Geometry: final body of the model. Coordinates: model frame, mm. Give positions to 0.01 mm unless a question says otherwise; leave off trailing zeros. Order: outer loops, then holes, each group sorted by start corner. A loop starts at its lowest first (then second) coordinate and runs counter-clockwise, first axis right, second up. Notation, with made-up numbers: M 29.25,-27 L 66.25,-27 A20 ccw 66.25,-9 Z; hole C 86.25,71 d5. An arc over 180 degrees is marked long. Use CSV: the item, a comma, the result in double quotes.
```python
from build123d import *

# Parameters (mm, degrees)
F0_W     = 2225
F0_H     = 100
F1_DEPTH = 125
F2_SIZE2 = 40
F2_SIZE  = 85


with BuildPart() as f1:
    # F0 (on Front) → F1 (new body)
    with BuildSketch(Plane.XZ):
        with Locations((-1112.5, -50)):
            Rectangle(F0_W, F0_H)
    extrude(amount=F1_DEPTH)

    # F2
    f2_edges = [f1.edges().sort_by_distance(p)[0] for p in [
        (-1112.5, -125, 0),
        (-2225, -62.5, 0),
    ]]
    f2_side = f1.faces().sort_by_distance((-1112.5, -62.5, 0))[0]
    chamfer(f2_edges, length=F2_SIZE, length2=F2_SIZE2, reference=f2_side)


solid = f1.part
```
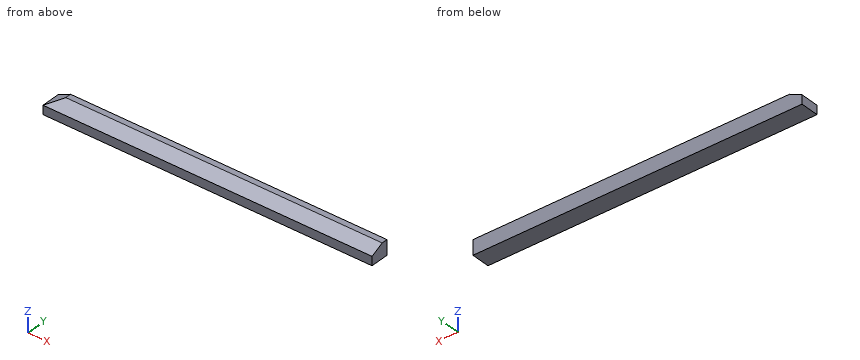
1. Section A-A, the plane x = -1465. Return the cut outline in (y, z).
Answer:
outline,"M -125,-100 L 0,-100 L 0,0 L -40,0 L -125,-40 Z"
2. Section B-B, the plane y = -87.5. Return the cut outline in (x, z), plus the area to 3 significant figures.
Answer:
outline,"M -2225,-100 L 0,-100 L 0,-22.35 L -2187.5,-22.35 L -2225,-40 Z"
area,"172,000 mm2"
3. Pin query (flat end, axial travel): pin 1 Ø1.5 at (x, y) = (-504.5, -109.5) entering from +Z; pin 2 Ø2 at (x, y) = (-1320.5, -83.5) entering from +Z. Return the tip coordinate at first contact, or that it passes through.
Answer:
pin 1,"z = -32.35"
pin 2,"z = -20"
4. Line query: line 1 (Z direction, x = -1782.5, y = -98); line 2 (Z direction, x = -882, y = -65); line 3 (Y direction, x = -1232.5, z = -25.5). Output: solid intervals per line, ascending.
Answer:
line 1,"-100 to -27.29"
line 2,"-100 to -11.76"
line 3,"-94.19 to 0"
